Part model, mm, in its own coordinate system. Give positions to 0.01 mm unless a question says otherwise; leave off trailing zeros. Write each loop counter-clockwise with the first axis right and the second up, starting at its lowest first coordinate (ties: lowest second). Pieces come first, ordered by that corner, then holes. Notation, with made-up numbers: (6.5, 32.25) - (28.5, 32.25) arc R15 ccw to (28.5, 55.25) - close; hole circle Ø8 at (19, 2). An arc over 180 degrees is marked (long way). Answer as a JSON object with one key per item and string values. Group by question number.
```python
from build123d import *

# Parameters (mm, degrees)
F0_R     = 8
F1_DEPTH = 10
F2_R     = 0.3
F3_DEPTH = 15
F4_R     = 1


with BuildPart() as f1:
    # F0 (on Top) → F1 (new body)
    with BuildSketch(Plane.XY):
        Circle(F0_R)
    extrude(amount=F1_DEPTH)

    # F2 (on face) → F3 (join)
    with BuildSketch(Plane(origin=(0, 0, 0), x_dir=(1, 0, 0), z_dir=(0, 0, -1))):
        with Locations((0, 3.868304)):
            Circle(F2_R)
        with Locations((0, -4.767918)):
            Circle(F2_R)
    extrude(amount=F3_DEPTH)

    # F4
    f4_edges = [f1.edges().sort_by_distance(p)[0] for p in [
        (-8, 0, 10),
        (-8, 0, 0),
    ]]
    fillet(f4_edges, radius=F4_R)


solid = f1.part
```
1) Drop flat-ended pins along their axis: P1, Ø1.5, axis at y = 4.5, z = 2.5, coming from the -X side; P2, Ø5, axis at y = -1, z = -12.5, coming from the +X side; P3, Ø1, axis at x = 4, z = 5.5, coming from the -Y side; P4, Ø7, axis at x = 2.5, y = -0.5, coming from the -Z side. Give the stop position or say it passes through.
2) Band-saw the part on A-A (y = 0). List the corners of the cut face in (x, z).
3) Band-saw the part on B-B (x = 0). List the corners of the cut face in (y, z).
4) Band-saw the part on C-C (z = -1.75). List the corners of the cut face in (x, y).
5) Probe line 1 (Z direction, x = -2, y = 0.25); line 2 (X direction, y = 4.75, z = -2.75); line 3 (X direction, y = -4, z = 8). List the from-to ranges inside material, lowest first.
Verdict:
{
 "1": {"P1": "x = -7.07", "P2": "through", "P3": "y = -7.19", "P4": "z = 0"},
 "2": {"outline": "(-8, 1) arc R1 ccw to (-7, 0) - (7, 0) arc R1 ccw to (8, 1) - (8, 9) arc R1 ccw to (7, 10) - (-7, 10) arc R1 ccw to (-8, 9) - close"},
 "3": {"outline": "(-8, 1) arc R1 ccw to (-7, 0) - (-4.17, 0) - (-4.17, -15) - (-3.57, -15) - (-3.57, 0) - (4.47, 0) - (4.47, -15) - (5.07, -15) - (5.07, 0) - (7, 0) arc R1 ccw to (8, 1) - (8, 9) arc R1 ccw to (7, 10) - (-7, 10) arc R1 ccw to (-8, 9) - close"},
 "4": {"outline": "circle Ø0.6 at (0, -3.87); circle Ø0.6 at (0, 4.77)"},
 "5": {"line 1": "0 to 10", "line 2": "-0.3 to 0.3", "line 3": "-6.93 to 6.93"}
}
